Geometry check sheet. Reference: the model listing, model coordinates, mm. A direction names the side the tool comes from. Round coordinates to 2 decimals unless told otherwise and drop trailing zeros. Write each loop counter-clockwise with the first axis right and the second up, starting at its lowest first coordinate (ties: lowest second). Pieces come first, ordered by that corner, then holes. Notation, with made-up numbers: M 45,-4.5 L 102,-4.5 A35 cw 102,33.5 Z; hole C 67,-23.75 d10. An arc over 180 degrees is marked long. Put each result on its own line as item: value. Start each with the question number.
(1) Gauge pin test, flat ends, axial feed: pin 1 (5 mm diameter, centred on x = 20, y = 10.5, fed in from +Z); pin 2 (1 mm diameter, centred on x = 79.5, y = 1, fed in from -Z); pin 3 (1 mm diameter, centred on x = 0.5, y = 1.5, fed in from +Z); pin 4 (8 mm diameter, centred on x = 53, z = 25.5, fed in from +Y). Record the tip position at first contact, or that the pin passes through.
(2) Section check A-A on z = 12. Record the cut outline in (x, y).
(3) Section check C-C on z = 43.5. Record the cut outline in (x, y), then the cut area to 3 significant figures.
(4) Section check B-B on y = 19. Record the cut outline in (x, z), then the cut area to 3 significant figures.
(5) Section check D-D on y = 26. Record the cut outline in (x, z).
(6) Tool access check on faces 4 (the flat face through (3.35, 1, 25)), 5 (the flat face through (1, 1, 40.64)), 6 (the flat face through (76.65, 1, 5)). Record the directions out of +Z, -Z, +X, -X, +Y, -Y that give a thin tool (end or side, any length) a straight path to the whole face; none if there is none.
(7) Material ranges on probe 1 along Y at (x, z) = (50.5, 5); probe 2 along X at (y, z) = (11, 38.5); probe 3 along X at (y, z) = (30, 3), recorded low to high.
(8) Mould release check, pull along Y, two halves, no side actions. Record for faces 1 (the flat face through (79, 1, 40.64)), 2 (the flat face through (65, 2, 28)), 3 (the flat face through (63, 0, 28)): pulls with the +Y half, pulls with the -Y half, needs draft (parallel to the pull), parting line crosses it, or undercut.
from build123d import *

# Parameters (mm, degrees)
F0_W     = 5
F0_H     = 10.16
F1_DEPTH = 2
F3_DEPTH = 55
F4_DEPTH = 55


with BuildPart() as f1:
    # F0 (on Front) → F1 (new body)
    with BuildSketch(Plane.XZ):
        Polygon((3.35, 0), (3.75, 0), (76.25, 0), (76.65, 0), (76.65, 10.16), (76.65, 20.32), (76.65, 30.48), (76.65, 40.64), (76.65, 55), (3.35, 55), (3.35, 40.64), (3.35, 30.48), (3.35, 20.32), (3.35, 10.16), align=None)
        with Locations((0.85, 15.24)):
            Rectangle(F0_W, F0_H)
        with Locations((79.15, 15.24)):
            Rectangle(F0_W, F0_H)
        with Locations((0.85, 35.56)):
            Rectangle(F0_W, F0_H)
        with Locations((79.15, 35.56)):
            Rectangle(F0_W, F0_H)
    extrude(amount=-F1_DEPTH)

    # F2 (on Top) → F3 (join)
    with BuildSketch(Plane.XY):
        with BuildLine():
            ThreePointArc((27.4464156413, 2), (30.3760816597, 29.8308767748), (54.1076163577, 15))
            ThreePointArc((54.1076163577, 15), (52.4384931326, 7.7684653019), (47.7688170742, 2))
            Line((47.7688170742, 2), (49.3229908716, 2))
            ThreePointArc((49.3229908716, 2), (53.5961912472, 7.8855447852), (55.1076163577, 15))
            ThreePointArc((55.1076163577, 15), (30.4931611429, 30.9885748895), (25.8922418439, 2))
            Line((25.8922418439, 2), (27.4464156413, 2))
        make_face()
    extrude(amount=F3_DEPTH)

    # F2 (on Top) → F4 (cut)
    with BuildSketch(Plane.XY):
        with BuildLine():
            Line((37.6076163577, 2), (27.4464156413, 2))
            ThreePointArc((27.4464156413, 2), (29.0315826838, 0.9038428491), (30.7337528153, 0))
            Line((30.7337528153, 0), (37.6076163577, 0))
            Line((37.6076163577, 0), (44.4814799001, 0))
            ThreePointArc((44.4814799001, 0), (46.1836500316, 0.9038428491), (47.7688170742, 2))
            Line((47.7688170742, 2), (37.6076163577, 2))
        make_face()
    extrude(amount=F4_DEPTH, mode=Mode.SUBTRACT)


solid = f1.part
Answers follow:
1. pin 1: stops at z = 55
1. pin 2: stops at z = 10.16
1. pin 3: stops at z = 40.64
1. pin 4: stops at y = 28.28
2. outline: M -1.65,0 L 30.73,0 A16.5 cw long 44.48,0 L 81.65,0 L 81.65,2 L 49.32,2 A17.5 ccw long 25.89,2 L -1.65,2 Z
3. outline: M 3.35,0 L 30.73,0 A16.5 cw long 44.48,0 L 76.65,0 L 76.65,2 L 49.32,2 A17.5 ccw long 25.89,2 L 3.35,2 Z
3. area: 195 mm^2
4. outline: M 20.57,0 L 21.6,0 L 21.6,55 L 20.57,55 Z; M 53.62,0 L 54.64,0 L 54.64,55 L 53.62,55 Z
4. area: 113 mm^2
5. outline: M 24,0 L 25.31,0 L 25.31,55 L 24,55 Z; M 49.91,0 L 51.22,0 L 51.22,55 L 49.91,55 Z
6. face 4: -X, +Y, -Y
6. face 5: +Z, -X, +Y, -Y
6. face 6: -Z, +X, +Y, -Y
7. probe 1: y = 0 to 2, 3.17 to 4.7, 25.3 to 26.83
7. probe 2: x = 20.57 to 21.6, 53.62 to 54.64
7. probe 3: x = 28.59 to 30.73, 44.48 to 46.62
8. face 1: needs draft
8. face 2: undercut
8. face 3: pulls with the -Y half
